Could you check a few things on this model? Use its own coordinates, in mm. Give positions to 0.01 mm unless a question says otherwise; leave off trailing zeros. Order: outer loops, then holes, each group sorted by start corner. A loop starts at its lowest first (then second) coordinate and runs counter-clockwise, first axis right, second up. Notation, with made-up numbers: M 82.25,83 L 139.25,83 A20 ccw 139.25,95 Z; hole C 20.5,23.5 d3. An arc over 180 degrees is marked long. Use a Markdown table: item, result. Add a question column.
```python
from build123d import *

# Parameters (mm, degrees)
SKIZZE1_W                       = 20
SKIZZE1_H                       = 40
AUFSATZ_LINEAR_AUSTRAGEN1_DEPTH = 300
SCHNITT_LINEAR_AUSTRAGEN1_DEPTH = 304.315017762
SKIZZE3_R                       = 3
SCHNITT_LINEAR_AUSTRAGEN2_DEPTH = 304.315017762


with BuildPart() as part:
    # Skizze1 → Aufsatz-Linear austragen1 (new body)
    with BuildSketch(Plane(origin=(0, 0, 0), x_dir=(1, 0, 0), z_dir=(0, 1, 0))):
        with Locations((10, 20)):
            Rectangle(SKIZZE1_W, SKIZZE1_H)
    extrude(amount=AUFSATZ_LINEAR_AUSTRAGEN1_DEPTH)

    # Skizze2 → Schnitt-Linear austragen1 (cut, through all)
    with BuildSketch(Plane(origin=(0, 300, 0), x_dir=(1, 0, 0), z_dir=(0, 1, 0))):
        Polygon((3, 30), (0, 33), (0, 27), align=None)
        Polygon((13, 40), (7, 40), (10, 37), align=None)
        Polygon((20, 27), (20, 33), (17, 30), align=None)
        Polygon((13, 20), (10, 17), (7, 20), align=None)
        Polygon((7, 20), (10, 23), (13, 20), align=None)
        Polygon((20, 7), (20, 13), (17, 10), align=None)
        Polygon((3, 10), (0, 13), (0, 7), align=None)
        Polygon((10, 3), (7, 0), (13, 0), align=None)
    extrude(amount=-SCHNITT_LINEAR_AUSTRAGEN1_DEPTH, mode=Mode.SUBTRACT)

    # Skizze3 → Schnitt-Linear austragen2 (cut, through all)
    with BuildSketch(Plane.XZ):
        with Locations(Location((10, -10, 0), (0, 0, 270))):
            Circle(SKIZZE3_R)
        with Locations(Location((10, -30, 0), (0, 0, 90))):
            Circle(SKIZZE3_R)
    extrude(amount=-SCHNITT_LINEAR_AUSTRAGEN2_DEPTH, mode=Mode.SUBTRACT)


solid = part.part
```
1) We'd pull the mould along Z, two halves only. Please class faces 1 (the face through (10, 148, -33)), 2 (the face through (3, 148, -40)), 3 (the face through (20, 148, -20)): pulls with the +Z half, pulls with the -Z half, needs draft (parallel to the pull), parting line crosses it, or undercut.
2) Suppose I cut it at A-A on y = 273. Please give me the cut outline in (x, z).
3) Please list where these lines run through material, in increasing order: line 1 (X direction, y = 113, z = -10); line 2 (Z direction, x = 10.25, y = 154); line 3 (Z direction, x = 1, y = 68). Write a range as from..to.
4) For pin 1 (1.5 mm diameter, centred on x = 10.5, y = 51.5, fed in from -Z); pin 2 (3.5 mm diameter, centred on x = 10, z = -30, fed in from -Y), each with a flat end and sliding along its axis, tell me the tip position at first contact or that it passes through.
Values found:
| question | item | result |
|---|---|---|
| 1 | face 1 | undercut |
| 1 | face 2 | pulls with the -Z half |
| 1 | face 3 | needs draft |
| 2 | outline | M 0,-40 L 7,-40 L 10,-37 L 13,-40 L 20,-40 L 20,-33 L 17,-30 L 20,-27 L 20,-13 L 17,-10 L 20,-7 L 20,0 L 13,0 L 10,-3 L 7,0 L 0,0 L 0,-7 L 3,-10 L 0,-13 L 0,-27 L 3,-30 L 0,-33 Z; hole C 10,-30 d6; hole M 7,-20 L 10,-23 L 13,-20 L 10,-17 Z; hole C 10,-10 d6 |
| 3 | line 1 | x = 3..7, 13..17 |
| 3 | line 2 | z = -37.25..-32.99, -27.01..-22.75, -17.25..-12.99, -7.01..-2.75 |
| 3 | line 3 | z = -40..-32, -28..-12, -8..0 |
| 4 | pin 1 | stops at z = -38.25 |
| 4 | pin 2 | passes through |
